Model file for the job. Use its own axes, mm. Round coordinates to 2 decimals unless told otherwise and drop trailing zeros. Loops run counter-clockwise (first coordinate to the right, second up) from the corner with the lowest first, then second, coordinate; pieces in that order, holes last.
Autodesk Inventor part; units mm, degrees
sketch "スケッチ1" plane through (0, 0, 0) normal (0, 0, 1) x (1, 0, 0)
  line L0 (-10, -10) -> (10, -10)
  line L1 (10, -10) -> (10, 10)
  line L2 (10, 10) -> (-10, 10)
  line L3 (-10, 10) -> (-10, -10)
  line L4 (-10, -10) -> (10, 10) construction
  line L5 (10, -10) -> (-10, 10) construction
  point P0 (0, 0)
  dimension "d0" = 20
  dimension "d1" = 20
extrude "押し出し1" add sketch "スケッチ1" along normal blind 1.6
sketch "スケッチ2" plane through (0, 0, 0) normal (0, 0, 1) x (1, 0, 0)
  circle A0 centre (-6.1, 7) radius 0.75
  circle A1 centre (6.1, 7) radius 0.75
  point P0 (0, 0)
  dimension "d9" = 1.5
  dimension "d10" = 7
  dimension "d11" = 6.1
  dimension "d14" = 1.5
  dimension "d15" = 12.2
extrude "押し出し2" cut sketch "スケッチ2" along normal blind 1.6
sketch "スケッチ3" plane through (0, 0, 0) normal (0, 0, 1) x (1, 0, 0)
  circle A0 centre (-6.1, 0) radius 0.5
  circle A1 centre (6.1, 0) radius 0.5
  point P0 (0, 0)
  dimension "d16" = 1
  dimension "d17" = 6.1
  dimension "d18" = 1
  dimension "d19" = 6.1
extrude "押し出し3" cut sketch "スケッチ3" along normal blind 1.6
sketch "スケッチ4" plane through (0, 0, 0) normal (0, 0, 1) x (1, 0, 0)
  circle A0 centre (0, 0) radius 1.5
  dimension "d22" = 3
extrude "押し出し4" cut sketch "スケッチ4" along normal blind 3
equation "\"d23\" = d22"
properties part number "HbBatteryPcb02" material "ABS プラスチック"
Q1. Slice it at C-C on x = 0. Give the cut face in (y, z).
Q2. Slice it at A-A on x = -6.1. Give the cut face in (y, z).
Q3. Flat gauge pin, fed straight in: P1, Ø2.5, axis at x = 0, y = 0, coming from the -Z side. Where does the tip first touch, or does it go through?
Q4. Probe line 1 (Y direction, x = 6.1, z = 0.9); line 2 (Y direction, x = 0, z = 0.5); line 3 (X direction, y = 1, z = 1.25). List the from-to ranges inside material, lowest first.
Q5. Slice it at B-B on y = 7. Give the cut face in (x, z), plus the area to 3 significant figures.
Q6. Pull direction Y, two halves, no side cores. Call faces 1 (the face through (0, 10, 1)), 2 (the face through (6.79, 7.29, 0.79)), 3 (the face through (10, 0, 1)): pulls with the +Y half, pulls with the -Y half, needs draft (parallel to the pull), parting line crosses it, or undercut.
Q7. Slice it at D-D on z = 1.05. Give the cut face in (x, y).
Reply:
1. outline: (-10, 0) - (-1.5, 0) - (-1.5, 1.6) - (-10, 1.6) - close; (1.5, 0) - (10, 0) - (10, 1.6) - (1.5, 1.6) - close
2. outline: (-10, 0) - (-0.5, 0) - (-0.5, 1.6) - (-10, 1.6) - close; (0.5, 0) - (6.25, 0) - (6.25, 1.6) - (0.5, 1.6) - close; (7.75, 0) - (10, 0) - (10, 1.6) - (7.75, 1.6) - close
3. P1: passes through
4. line 1: y = -10 to -0.5, 0.5 to 6.25, 7.75 to 10
4. line 2: y = -10 to -1.5, 1.5 to 10
4. line 3: x = -10 to -1.12, 1.12 to 10
5. outline: (-10, 0) - (-6.85, 0) - (-6.85, 1.6) - (-10, 1.6) - close; (-5.35, 0) - (5.35, 0) - (5.35, 1.6) - (-5.35, 1.6) - close; (6.85, 0) - (10, 0) - (10, 1.6) - (6.85, 1.6) - close
5. area: 27.2 mm2
6. face 1: pulls with the +Y half
6. face 2: undercut
6. face 3: needs draft
7. outline: (-10, -10) - (10, -10) - (10, 10) - (-10, 10) - close; hole circle Ø1.5 at (-6.1, 7); hole circle Ø1 at (-6.1, 0); hole circle Ø3 at (0, 0); hole circle Ø1.5 at (6.1, 7); hole circle Ø1 at (6.1, 0)
